```python
from build123d import *

# Parameters (mm, degrees)
F1_DEPTH = 63.5
F2_DEPTH = 7.9375
F0_W     = 25.4
F0_H     = 19.05
F3_DEPTH = 25.4
F5_R     = 6.35


with BuildPart() as f1:
    # F0 (on Front) → F1 (new body, symmetric)
    with BuildSketch(Plane.XZ):
        Polygon((-41.275, -9.525), (41.275, -9.525), (41.275, 9.525), (22.225, 9.525), (-41.275, 9.525), align=None)
    extrude(amount=F1_DEPTH, both=True)

    # F0 (on Front) → F2 (join, symmetric)
    with BuildSketch(Plane.XZ):
        with BuildLine():
            add(Edge.make_bspline(
                [(-41.275, 9.525), (-40.6536376941, 44.0692058558), (5.3086092688, 60.1907536905), (55.0853842739, 61.8641209915)],
                knots=[0, 0, 0, 0, 109.9854236751, 109.9854236751, 109.9854236751, 109.9854236751], degree=3))
            Line((-41.275, 9.525), (22.225, 9.525))
            Line((22.225, 9.525), (22.225, 27.0002))
            ThreePointArc((22.225, 27.0002), (31.7348241278, 50.9548333803), (55.0853842739, 61.8641209915))
        make_face()
    extrude(amount=F2_DEPTH, both=True)

    # F0 (on Front) → F3 (join, symmetric)
    with BuildSketch(Plane.XZ):
        with BuildLine():
            Line((22.225, 9.525), (41.275, 9.525))
            Line((41.275, 9.525), (41.275, 27.0002))
            ThreePointArc((41.275, 27.0002), (45.9246798487, 38.2255201513), (57.15, 42.8752))
            Line((57.15, 42.8752), (60.325, 42.8752))
            Line((60.325, 42.8752), (60.325, 61.9252))
            Line((60.325, 61.9252), (57.15, 61.9252))
            add(Edge.make_bspline(
                [(55.0853842739, 61.8641209915), (55.7728982919, 61.8872334466), (56.4611400065, 61.9075896253), (57.15, 61.9252)],
                knots=[109.9854236751, 109.9854236751, 109.9854236751, 109.9854236751, 111.5045361635, 111.5045361635, 111.5045361635, 111.5045361635], degree=3))
            ThreePointArc((55.0853842739, 61.8641209915), (31.7348241278, 50.9548333803), (22.225, 27.0002))
            Line((22.225, 27.0002), (22.225, 9.525))
        make_face()
        with Locations((73.025, 52.4002)):
            Rectangle(F0_W, F0_H)
    extrude(amount=F3_DEPTH, both=True)

    # F0 (on Front) → F4 (revolve)
    with BuildSketch(Plane.XZ):
        Polygon((85.725, 61.9252), (85.725, 42.8752), (85.725, 38.1), (111.125, 38.1), (111.125, 66.675), (85.725, 66.675), align=None)
    revolve(axis=Axis((85.725, 0, 52.3875), (0, 0, -1)))

    # F5
    f5_edges = [f1.edges().sort_by_distance(p)[0] for p in [
        (-41.275, -63.5, 0),
        (41.275, -63.5, 0),
        (41.275, 63.5, 0),
        (-41.275, 63.5, 0),
    ]]
    fillet(f5_edges, radius=F5_R)


solid = f1.part
```
Verification items for the finished model (mm, model axes). A direction names the side the tool comes from. Round coordinates to 2 decimals unless told otherwise and drop trailing zeros. Loops run counter-clockwise (first coordinate to the right, second up) from the corner with the lowest first, then second, coordinate; pieces in that order, holes last. Notation, with made-up numbers: (62.25, 64.25) -> (104.25, 64.25) arc R18 cw to (104.25, 92.25) -> close; hole circle Ø6 at (75, 26.25). An arc over 180 degrees is marked (long way). Answer as a JSON object with one key per item and string values.
Q1. Draft check along X on faces 1 (the flat face through (60, -2, 61.925)), 2 (the flat face through (-41.275, -1, 0)), 3 (the cylindrical face through (45.8, -0.4, 38.1)). Enter one of: pulls with the +X half, pulls with the -X half, needs draft (parallel to the pull), parting line crosses it, or undercut.
Data:
{"face 1": "needs draft", "face 2": "pulls with the -X half", "face 3": "undercut"}
Q2. Scan lines: line 1 (Y direction, x = 41, z = 37); line 2 (Z direction, x = -13, y = 58.5) (3 decimals); line 3 (Z direction, x = 82, y = -4.5) (3 decimals). Record each from-to range of solid material in increasing order. Write a range as from..to.
Data:
{"line 1": "y = -25.4..25.4", "line 2": "z = -9.525..9.525", "line 3": "z = 38.1..66.675"}
Q3. Section check A-A (y = -44.5). Record the boundary of the cut face in (x, z) (3 decimals).
Data:
{"outline": "(-41.275, -9.525) -> (41.275, -9.525) -> (41.275, 9.525) -> (-41.275, 9.525) -> close"}
Q4. Go/stop test with flat-tipped pins: P1, Ø15.5, axis at x = 8, z = 41.5, coming from the +Y side; P2, Ø14.5, axis at x = 69, y = 6.5, coming from the -Z side; P3, Ø3, axis at y = -3, z = 45, coming from the -X side. Record where each tip stops, or that it passes through.
Data:
{"P1": "stops at y = 7.94", "P2": "stops at z = 38.1", "P3": "stops at x = -19.73"}
Q5. Access from +Z, -Z, +X, -X, +Y, -Y to the whole of each face (thin tool, end or side, straight path). Record for faces 4 (the flat face through (1, -36, 9.525)), 5 (the flat face through (-3, 7.938, 30)), 6 (the flat face through (86, 0, 38.1)), 7 (the flat face through (46, 25.4, 42)).
Data:
{"face 4": "+Z, -X, -Y", "face 5": "+Z, -X, +Y", "face 6": "-Z, +X, +Y, -Y", "face 7": "+Z, +X, -X, +Y"}
